Geometry check sheet. Reference: the model listing, model coordinates, mm. A direction names the side the tool comes from. Give positions to 0.01 mm unless a question says otherwise; leave off trailing zeros. Write each loop counter-clockwise with the first axis right and the second up, starting at its lowest first coordinate (ties: lowest second). Pieces come first, ordered by that corner, then holes.
(1) Cross-section at B-B (z = 79). Record the boundary of the cut face in (x, y).
(2) Cross-section at C-C (z = 279). Record the boundary of the cut face in (x, y), and give its area (3 significant figures).
(3) Thickness scan on line 1 along Z through (x, y) = (41, 3); line 2 along X through (y, z) = (38, -80); line 3 along X through (y, z) = (2.5, 99). Record the ranges inside material, lowest first.
(4) Mould release check, pull along Z, two halves, no side actions. Record for faces 1 (the cylindrical face through (38.07, 1.97, 241.31)), 2 (the flat face through (40, 2, -100)), 3 (the flat face through (80, 20, 132)): +Z half, -Z half, draft (parallel to the pull), parting line (faces both ways), or undercut.
(5) Cross-section at A-A (x = 41). Record the boundary of the cut face in (y, z), and give its area (3 significant figures).
(6) Depth check by flat-ended pin: P1, Ø4.5, axis at x = 60, z = 124, coming from the +Y side; P2, Ø5, axis at x = 68, z = 12, coming from the +Y side. Enter the tip coordinate at first touch or a pass-through.
(7) Tool access check on faces 4 (the flat face through (4, 22, 132)), 5 (the flat face through (40, 2, 358)). Record the directions out of +Z, -Z, +X, -X, +Y, -Y that give a thin tool (end or side, any length) a straight path to the whole face; none if there is none.
```python
from build123d import *

# Parameters (mm, degrees)
EXTRUDE_1_DEPTH             = 298
SKETCH_2_R                  = 22.5
CUT_EXTRUDE_1_DEPTH         = 312.133411899
HOLE_WIZARD_M62_D           = 5
HOLE_WIZARD_M62_DEPTH       = 17
HOLE_WIZARD_M62_CSINK_D     = 6.05
HOLE_WIZARD_M62_CSINK_ANGLE = 120
HOLE_WIZARD_M62_TIP         = 1.502151548
HOLE_WIZARD_M42_D           = 4.5
HOLE_WIZARD_M42_DEPTH       = 5
HOLE_WIZARD_M42_TIP         = 1.351936393
HOLE_WIZARD_M63_D           = 5
HOLE_WIZARD_M63_DEPTH       = 17
HOLE_WIZARD_M63_CSINK_D     = 6.05
HOLE_WIZARD_M63_CSINK_ANGLE = 120
HOLE_WIZARD_M63_TIP         = 1.502151548
EXTRUDE_2_DEPTH             = 60
EXTRUDE_3_DEPTH             = 100
HOLE_WIZARD_M61_D           = 6.6
HOLE_WIZARD_M61_DEPTH       = 5
HOLE_WIZARD_M61_TIP         = 1.982840043


with BuildPart() as part:
    # Эскиз1 → Бобышка-Вытянуть1 (new body)
    with BuildSketch(Plane.XY):
        Polygon((0, 0), (0, 40), (4, 40), (4, 4), (76, 4), (76, 40), (80, 40), (80, 0), align=None)
    extrude(amount=EXTRUDE_1_DEPTH)

    # Эскиз2 → Вырез-Вытянуть1 (cut, through all)
    with BuildSketch(Plane.XZ):
        with Locations((41, 219)):
            Circle(SKETCH_2_R)
        with Locations((41, 79)):
            Circle(SKETCH_2_R)
    extrude(amount=-CUT_EXTRUDE_1_DEPTH, mode=Mode.SUBTRACT)

    # Отверстие обработанное метчиком M62
    with Locations(Plane(origin=(0, 4, 0), x_dir=(-1, 0, 0), z_dir=(0, 1, 0))):
        with Locations((-21.554563517, 98.445436483), (-21.554563517, 59.554563517), (-60.445436483, 59.554563517), (-60.445436483, 98.445436483), (-60.445436483, 199.554563517), (-60.445436483, 238.445436483), (-21.554563517, 238.445436483), (-21.554563517, 199.554563517)):
            CounterSinkHole(HOLE_WIZARD_M62_D / 2, HOLE_WIZARD_M62_CSINK_D / 2, depth=HOLE_WIZARD_M62_DEPTH, counter_sink_angle=HOLE_WIZARD_M62_CSINK_ANGLE)
            with Locations((0, 0, -(HOLE_WIZARD_M62_DEPTH + HOLE_WIZARD_M62_TIP / 2))):  # 118° drill point
                Cone(0, HOLE_WIZARD_M62_D / 2, HOLE_WIZARD_M62_TIP, mode=Mode.SUBTRACT)

    # Отверстие с зазором M42
    with Locations(Plane(origin=(80, 0, 0), x_dir=(0, 0, -1), z_dir=(1, 0, 0))):
        with Locations((-288, 34), (-30, 34), (-268, 34), (-10, 34), (-288, 14), (-30, 14), (-268, 14), (-10, 14)):
            Hole(HOLE_WIZARD_M42_D / 2, depth=HOLE_WIZARD_M42_DEPTH)
            with Locations((0, 0, -(HOLE_WIZARD_M42_DEPTH + HOLE_WIZARD_M42_TIP / 2))):  # 118° drill point
                Cone(0, HOLE_WIZARD_M42_D / 2, HOLE_WIZARD_M42_TIP, mode=Mode.SUBTRACT)

    # Отверстие обработанное метчиком M63
    with Locations(Plane.XZ):
        with Locations((20, 124), (20, 174), (60, 174), (60, 124)):
            CounterSinkHole(HOLE_WIZARD_M63_D / 2, HOLE_WIZARD_M63_CSINK_D / 2, depth=HOLE_WIZARD_M63_DEPTH, counter_sink_angle=HOLE_WIZARD_M63_CSINK_ANGLE)
            with Locations((0, 0, -(HOLE_WIZARD_M63_DEPTH + HOLE_WIZARD_M63_TIP / 2))):  # 118° drill point
                Cone(0, HOLE_WIZARD_M63_D / 2, HOLE_WIZARD_M63_TIP, mode=Mode.SUBTRACT)

    # Эскиз15 → Бобышка-Вытянуть2 (add)
    with BuildSketch(Plane.XY.offset(298)):
        Polygon((4, 4), (4, 40), (0, 40), (0, 0), (80, 0), (80, 40), (76, 40), (76, 4), align=None)
    extrude(amount=EXTRUDE_2_DEPTH)

    # Эскиз17 → Бобышка-Вытянуть3 (add)
    with BuildSketch(Plane(origin=(0, 0, 0), x_dir=(-1, 0, 0), z_dir=(0, 0, -1))):
        Polygon((-4, 4), (-4, 40), (0, 40), (0, 0), (-80, 0), (-80, 40), (-76, 40), (-76, 4), align=None)
    extrude(amount=EXTRUDE_3_DEPTH)

    # Отверстие с зазором M61
    with Locations(Plane(origin=(0, 4, 0), x_dir=(-1, 0, 0), z_dir=(0, 1, 0))):
        with Locations((-20, 338), (-60, 338), (-60, -80), (-20, -80)):
            Hole(HOLE_WIZARD_M61_D / 2, depth=HOLE_WIZARD_M61_DEPTH)
            with Locations((0, 0, -(HOLE_WIZARD_M61_DEPTH + HOLE_WIZARD_M61_TIP / 2))):  # 118° drill point
                Cone(0, HOLE_WIZARD_M61_D / 2, HOLE_WIZARD_M61_TIP, mode=Mode.SUBTRACT)


solid = part.part
```
Reply:
1. outline: (0, 0) - (18.5, 0) - (18.5, 4) - (4, 4) - (4, 40) - (0, 40) - close; (63.5, 0) - (80, 0) - (80, 40) - (76, 40) - (76, 4) - (63.5, 4) - close
2. outline: (0, 0) - (80, 0) - (80, 40) - (76, 40) - (76, 4) - (4, 4) - (4, 40) - (0, 40) - close
2. area: 608 mm2
3. line 1: z = -100 to 56.5, 101.5 to 196.5, 241.5 to 358
3. line 2: x = 0 to 4, 76 to 80
3. line 3: x = 0 to 19.12, 23.99 to 30.69, 51.31 to 58.01, 62.88 to 80
4. face 1: undercut
4. face 2: -Z half
4. face 3: draft
5. outline: (0, -100) - (4, -100) - (4, 56.5) - (0, 56.5) - close; (0, 101.5) - (4, 101.5) - (4, 196.5) - (0, 196.5) - close; (0, 241.5) - (4, 241.5) - (4, 358) - (0, 358) - close
5. area: 1,470 mm2
6. P1: passes through
6. P2: stops at y = 4
7. face 4: +Z, -Z, +Y
7. face 5: +Z, +X, -X, +Y, -Y
